```python
from build123d import *

# Parameters (mm, degrees)
BOSS_EXTRUDE1_DEPTH = 12.7
SKETCH3_R           = 1.27
BOSS_EXTRUDE2_DEPTH = 12.7
CUT_EXTRUDE6_START  = 13.462
CUT_EXTRUDE6_DEPTH  = 13.462
FILLET2_R           = 2.54
FILLET3_R           = 2.54
FILLET4_R           = 2.54
FILLET5_R           = 2.54
FILLET6_R           = 1


with BuildPart() as part:
    # Sketch1 → Boss-Extrude1 (new body)
    with BuildSketch(Plane.XY):
        Polygon((-5.08, -5.08), (-5.08, 11.43), (0, 11.43), (0, 0), (15.24, 0), (15.24, 11.43), (20.32, 11.43), (20.32, -5.08), align=None)
    extrude(amount=BOSS_EXTRUDE1_DEPTH)

    # Sketch3 → Boss-Extrude2 (add)
    with BuildSketch(Plane.XY.offset(12.7)):
        with BuildLine():
            Line((-5.08, 5.08), (-5.08, 12.532978233))
            ThreePointArc((-5.08, 12.532978233), (-9.961764292, 13.516716003), (-5.842, 10.719055412))
            Line((-5.842, 10.719055412), (-5.842, 5.08))
            Line((-5.842, 5.08), (-5.08, 5.08))
        make_face()
        with Locations((-7.62, 12.532978233)):
            Circle(SKETCH3_R, mode=Mode.SUBTRACT)
    boss_extrude2 = extrude(amount=-BOSS_EXTRUDE2_DEPTH)

    # Sketch9 → Cut-Extrude6 (cut)
    with BuildSketch(Plane.XY.offset(10.033).offset(CUT_EXTRUDE6_START)):
        with BuildLine():
            Line((-5.08, 12.532978233), (-5.08, 11.43))
            Line((-5.08, 11.43), (-5.842, 10.719055412))
            ThreePointArc((-5.842, 10.719055412), (-9.961764292, 13.516716003), (-5.08, 12.532978233))
        make_face()
        with BuildLine():
            Line((21.082, 10.719055412), (20.32, 11.43))
            Line((20.32, 11.43), (20.32, 12.532978233))
            ThreePointArc((20.32, 12.532978233), (25.201764292, 13.516716003), (21.082, 10.719055412))
        make_face()
    cut_extrude6 = extrude(amount=-CUT_EXTRUDE6_DEPTH, mode=Mode.SUBTRACT)

    # Fillet2
    fillet2_edges = [part.edges().sort_by_distance(p)[0] for p in [
        (15.24, 11.43, 6.35),
        (0, 11.43, 6.35),
    ]]
    fillet(fillet2_edges, radius=FILLET2_R)

    # Fillet3
    fillet3_edges = [part.edges().sort_by_distance(p)[0] for p in [
        (0, 0, 6.35),
        (15.24, 0, 6.35),
    ]]
    fillet(fillet3_edges, radius=FILLET3_R)

    # Mirror1: Boss-Extrude2, Cut-Extrude6 across plane
    add(boss_extrude2.mirror(Plane(origin=(7.62, 0, 0), x_dir=(0, 0, 1), z_dir=(1, 0, 0))))
    add(cut_extrude6.mirror(Plane(origin=(7.62, 0, 0), x_dir=(0, 0, 1), z_dir=(1, 0, 0))), mode=Mode.SUBTRACT)

    # Mirror3: Cut-Extrude6 across plane
    add(cut_extrude6.mirror(Plane.XY.offset(6.35)), mode=Mode.SUBTRACT)

    # Fillet4
    # the kernel refuses this fillet: 2.54 mm, written as the material it adds along each edge
    with BuildSketch(Plane(origin=(20.32, 11.43, 10.033), x_dir=(-1, 0, 0), z_dir=(0, 0, -1)), Plane(origin=(-5.08, 11.43, 2.667), x_dir=(1, 0, 0), z_dir=(0, 0, 1))) as fillet4_piece_1:
        with BuildLine():
            CenterArc((2.332511513, 2.54), FILLET4_R, 196.432066058, 73.567933942)
            Line((-0.103744244, 1.821489116), (-0.347369819, 1.749638028))
            ThreePointArc((-0.347369819, 1.749638028), (-0.254, 1.102978233), (-0.254, 0))
            Line((-0.254, 0), (0, -0.254))
            Line((0, -0.254), (2.332511513, -0.254))
            Line((2.332511513, -0.254), (2.332511513, 0))
        make_face()
    extrude(amount=7.366)
    with BuildSketch(Plane(origin=(20.32, 5.08, 12.7), x_dir=(0, -1, 0), z_dir=(0, 0, -1))) as fillet4_piece_2:
        with BuildLine():
            CenterArc((1.813922821, -2.54), FILLET4_R, 90, 45.572995999)
            Line((0, -0.762), (0, 0))
            Line((0, 0), (1.813922821, 0))
        make_face()
    extrude(amount=12.7)
    with BuildSketch(Plane(origin=(-5.08, 5.08, 12.7), x_dir=(-1, 0, 0), z_dir=(0, 0, -1))) as fillet4_piece_3:
        with BuildLine():
            CenterArc((2.54, -1.813922821), FILLET4_R, 134.427004001, 45.572995999)
            Line((0, -1.813922821), (0, 0))
            Line((0, 0), (0.762, 0))
        make_face()
    extrude(amount=12.7)
    # the kernel refuses this fillet: 2.54 mm, written as the material it takes off along each edge
    with BuildSketch(Plane(origin=(-5.842, 10.719055412, 15.457445582), x_dir=(0.7311775057890088, 0.6821872580370908, 0), z_dir=(0, 0, -1)), Plane(origin=(-5.842, 10.719055412, 2.667), x_dir=(0.7311775057890088, 0.6821872580370908, 0), z_dir=(0, 0, -1))) as fillet4_2_piece_1:
        with BuildLine():
            CenterArc((1.104753168, 2.539228509), FILLET4_R, 223.014800445, 45.572995999)
            Line((-0.752437696, 0.806472873), (0, 0))
            Line((0, 0), (1.042154599, 0))
        make_face()
    extrude(amount=5.424445582, mode=Mode.SUBTRACT)
    with BuildSketch(Plane(origin=(21.082, 10.719055412, 2.667), x_dir=(-0.7311775057890088, 0.6821872580370906, 0), z_dir=(0, 0, -1))) as fillet4_2_piece_2:
        with BuildLine():
            CenterArc((1.104753168, -2.539228509), FILLET4_R, 91.412203555, 45.572995999)
            Line((-0.752437696, -0.806472873), (0, 0))
            Line((0, 0), (1.042154599, 0))
        make_face()
    extrude(amount=5.424445582, mode=Mode.SUBTRACT)
    with BuildSketch(Plane(origin=(21.082, 10.719055412, 15.457445582), x_dir=(0, -1, 0), z_dir=(0, 0, -1))) as fillet4_2_piece_3:
        with BuildLine():
            CenterArc((1.102978233, 2.54), FILLET4_R, 224.427004001, 45.572995999)
            Line((-0.710944588, 0.762), (0, 0))
            Line((0, 0), (1.102978233, 0))
        make_face()
    extrude(amount=5.424445582, mode=Mode.SUBTRACT)

    # Fillet5
    fillet5_edges = [part.edges().sort_by_distance(p)[0] for p in [
        (20.32, -5.08, 6.35),
        (-5.08, -5.08, 6.35),
        (-5.842, 5.08, 6.35),
        (21.082, 5.08, 6.35),
    ]]
    fillet(fillet5_edges, radius=FILLET5_R)

    # Fillet6
    fillet6_edges = [part.edges().sort_by_distance(p)[0] for p in [
        (-5.08, 11.43, 1.3335),
        (20.32, 11.43, 11.3665),
        (20.32, 11.43, 1.3335),
        (-5.08, 11.43, 11.3665),
    ]]
    fillet(fillet6_edges, radius=FILLET6_R)


solid = part.part
```
The model under review builds one solid part; all positions refer to its coordinate system, in mm. A direction names the side the tool comes from. Round coordinates to 2 decimals unless told otherwise and drop trailing zeros. Order: outer loops, then holes, each group sorted by start corner. A loop starts at its lowest first (then second) coordinate and runs counter-clockwise, first axis right, second up.
Item 1: Draft analysis for pull direction Y (two halves, no side actions). For faces 5 (the cylindrical face through (21.649, 12.914, 6.402)), 6 (the cylindrical face through (-4.356, -4.316, 6.439)), 7 (the cylindrical face through (20.34, 11.3, 11.39)), 8 (the flat face through (21.6, 11.8, 10.033)), state which applies: released by +Y, released by -Y, zero draft, split by the parting line, or undercut.
Working result:
face 5: undercut
face 6: released by -Y
face 7: released by +Y
face 8: zero draft
Item 2: Add section B-B, the plane x = 22.86. State the section outline as (y, z) points, and give its area (3 significant figures).
Working result:
outline: (9.99, 2.67) - (11.26, 2.67) - (11.26, 10.03) - (9.99, 10.03) - close; (13.8, 2.67) - (15.07, 2.67) - (15.07, 10.03) - (13.8, 10.03) - close
area: 18.7 mm2
Item 3: Add section C-C, the plane z = 1.25. State the section outline as (x, y) points, and give its area (3 significant figures).
Working result:
outline: (-5.84, 5.94) arc R2.54 ccw to (-5.46, 4.6) arc R2.54 cw to (-5.08, 3.27) - (-5.08, -2.54) arc R2.54 ccw to (-2.54, -5.08) - (17.78, -5.08) arc R2.54 ccw to (20.32, -2.54) - (20.32, 3.27) arc R2.54 cw to (20.7, 4.6) arc R2.54 ccw to (21.08, 5.94) - (21.08, 9.62) arc R2.54 ccw to (20.7, 10.96) arc R1 ccw to (19.85, 11.43) - (17.78, 11.43) arc R2.54 ccw to (15.24, 8.89) - (15.24, 2.54) arc R2.54 cw to (12.7, 0) - (2.54, 0) arc R2.54 cw to (0, 2.54) - (0, 8.89) arc R2.54 ccw to (-2.54, 11.43) - (-4.61, 11.43) arc R1 ccw to (-5.46, 10.96) arc R2.54 ccw to (-5.84, 9.62) - close
area: 252 mm2
Item 4: Add section A-A, the plane y = 8. State the section outline as (x, z) points.
Working result:
outline: (-5.84, 0) - (0, 0) - (0, 12.7) - (-5.84, 12.7) - close; (15.24, 0) - (21.08, 0) - (21.08, 12.7) - (15.24, 12.7) - close
Item 5: Add section D-D, the plane y = 12. State the section outline as (x, z) points, and give its area (3 significant figures).
Working result:
outline: (-10.1, 2.67) - (-8.77, 2.67) - (-8.77, 10.03) - (-10.1, 10.03) - close; (-6.47, 2.67) - (-4.35, 2.67) - (-4.35, 10.03) - (-6.47, 10.03) - close; (19.59, 2.67) - (21.71, 2.67) - (21.71, 10.03) - (19.59, 10.03) - close; (24.01, 2.67) - (25.34, 2.67) - (25.34, 10.03) - (24.01, 10.03) - close
area: 50.8 mm2
Item 6: To check wall thickness, follow probe 1 along Y at (x, z) = (22.86, 8); probe 2 along X at (y, z) = (2.75, 3.25); probe 3 along Y at (x, z) = (3, 1). State the ranges of each line that lie inside material, in increasing order.
Working result:
probe 1: y = 9.99 to 11.26, 13.8 to 15.07
probe 2: x = -5.08 to 0, 15.24 to 20.32
probe 3: y = -5.08 to 0
Item 7: For pin 1 (1.4 mm diameter, centred on y = 8.5, z = 4.5, fed in from -X); pin 2 (1 mm diameter, centred on y = 13, z = 10, fed in from +X); pin 3 (4 mm diameter, centred on x = 22.86, y = 12.53, fed in from +Z); pin 4 (1.5 mm diameter, centred on x = -1, z = 3.5, fed in from +Y), all flat-tipped, find the tip position at first contact; note any pin that passes through.
Working result:
pin 1: stops at x = -5.84
pin 2: stops at x = 25.4
pin 3: stops at z = 10.03
pin 4: stops at y = 11.3
Item 8: Machinability: for faces 1 (the flat face through (-8, 11, 10.033)), 2 (the cylindrical face through (-5.75, 10.3, 1.35)), 3 (the flat face through (19, 11.43, 2)), 4 (the flat face through (20.32, 0, 6)), which of the approach directions +Z, -Z, +X, -X, +Y, -Y give a long, thin tool a straight path to every point of the face, cutting with its end or side? Answer none if there is none.
Working result:
face 1: +Z, -X, +Y
face 2: -Z, -X, +Y
face 3: +Y
face 4: +Z, -Z, +X, -Y
